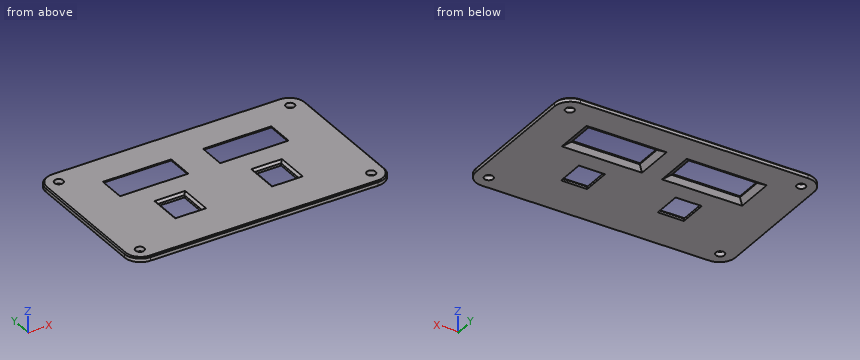
from build123d import *
from OCP.BRepFilletAPI import BRepFilletAPI_MakeChamfer

# Parameters (mm, degrees)
SKETCH1_R           = 1.9
BOSS_EXTRUDE1_DEPTH = 2
SKETCH6_W           = 11.5
SKETCH6_H           = 12.5
SKETCH6_W_2         = 30
SKETCH6_H_2         = 12
CUT_EXTRUDE2_DEPTH  = 2
CHAMFER4_SIZE       = 1
CHAMFER5_SIZE       = 1.5
CHAMFER5_SIZE2      = 2.598076211
CHAMFER6_SIZE       = 0.5


with BuildPart() as part:
    # Sketch1 → Boss-Extrude1 (new body)
    with BuildSketch(Plane.XY):
        with BuildLine():
            Line((-57, 27.5), (-57, -27.5))
            ThreePointArc((-57, -27.5), (-54.949747468, -32.449747468), (-50, -34.5))
            Line((-50, -34.5), (50, -34.5))
            ThreePointArc((50, -34.5), (54.949747468, -32.449747468), (57, -27.5))
            Line((57, -27.5), (57, 27.5))
            ThreePointArc((57, 27.5), (54.949747468, 32.449747468), (50, 34.5))
            Line((50, 34.5), (-50, 34.5))
            ThreePointArc((-50, 34.5), (-54.949747468, 32.449747468), (-57, 27.5))
        make_face()
        with Locations((-50.814035536, 28.314035536)):
            Circle(SKETCH1_R, mode=Mode.SUBTRACT)
        with Locations((50.814035536, 28.314035536)):
            Circle(SKETCH1_R, mode=Mode.SUBTRACT)
        with Locations((50.814035536, -28.314035536)):
            Circle(SKETCH1_R, mode=Mode.SUBTRACT)
        with Locations((-50.814035536, -28.314035536)):
            Circle(SKETCH1_R, mode=Mode.SUBTRACT)
    extrude(amount=BOSS_EXTRUDE1_DEPTH)

    # Sketch6 → Cut-Extrude2 (cut)
    with BuildSketch(Plane.XY.offset(2)):
        with Locations((-21.25, -9.5)):
            Rectangle(SKETCH6_W, SKETCH6_H)
        with Locations((21.25, -9.5)):
            Rectangle(SKETCH6_W, SKETCH6_H)
        with Locations((-22, 13.5)):
            Rectangle(SKETCH6_W_2, SKETCH6_H_2)
        with Locations((22, 13.5)):
            Rectangle(SKETCH6_W_2, SKETCH6_H_2)
    extrude(amount=-CUT_EXTRUDE2_DEPTH, mode=Mode.SUBTRACT)

    # Chamfer4
    chamfer4_edges = [part.edges().sort_by_distance(p)[0] for p in [
        (27, -9.5, 2),
        (21.25, -3.25, 2),
        (15.5, -9.5, 2),
        (21.25, -15.75, 2),
        (-15.5, -9.5, 2),
        (-21.25, -3.25, 2),
        (-27, -9.5, 2),
        (-21.25, -15.75, 2),
    ]]
    chamfer(chamfer4_edges, length=CHAMFER4_SIZE)

    # Chamfer5: one chamfer whose edges measure the first distance from different faces: ONE call of the kernel's chamfer builder (chamfer() names one face for all edges)
    chamfer5_edges_1 = [part.edges().sort_by_distance(p)[0] for p in [
        (-7, 13.5, 0),
    ]]
    chamfer5_side_1 = [part.faces().sort_by_distance(p)[0] for p in [
        (-7, 13.5, 1),
    ]]
    chamfer5_edges_2 = [part.edges().sort_by_distance(p)[0] for p in [
        (-22, 7.5, 0),
    ]]
    chamfer5_side_2 = [part.faces().sort_by_distance(p)[0] for p in [
        (-22, 7.5, 1),
    ]]
    chamfer5_edges_3 = [part.edges().sort_by_distance(p)[0] for p in [
        (-37, 13.5, 0),
    ]]
    chamfer5_side_3 = [part.faces().sort_by_distance(p)[0] for p in [
        (-37, 13.5, 1),
    ]]
    chamfer5_edges_4 = [part.edges().sort_by_distance(p)[0] for p in [
        (-22, 19.5, 0),
    ]]
    chamfer5_side_4 = [part.faces().sort_by_distance(p)[0] for p in [
        (-22, 19.5, 1),
    ]]
    chamfer5_edges_5 = [part.edges().sort_by_distance(p)[0] for p in [
        (37, 13.5, 0),
    ]]
    chamfer5_side_5 = [part.faces().sort_by_distance(p)[0] for p in [
        (37, 13.5, 1),
    ]]
    chamfer5_edges_6 = [part.edges().sort_by_distance(p)[0] for p in [
        (22, 7.5, 0),
    ]]
    chamfer5_side_6 = [part.faces().sort_by_distance(p)[0] for p in [
        (22, 7.5, 1),
    ]]
    chamfer5_edges_7 = [part.edges().sort_by_distance(p)[0] for p in [
        (7, 13.5, 0),
    ]]
    chamfer5_side_7 = [part.faces().sort_by_distance(p)[0] for p in [
        (7, 13.5, 1),
    ]]
    chamfer5_edges_8 = [part.edges().sort_by_distance(p)[0] for p in [
        (22, 19.5, 0),
    ]]
    chamfer5_side_8 = [part.faces().sort_by_distance(p)[0] for p in [
        (22, 19.5, 1),
    ]]
    chamfer5 = BRepFilletAPI_MakeChamfer(part.part.solid().wrapped)
    for e in chamfer5_edges_1:
        chamfer5.Add(CHAMFER5_SIZE, CHAMFER5_SIZE2, e.wrapped, chamfer5_side_1[0].wrapped)  # the first distance lies on this face
    for e in chamfer5_edges_2:
        chamfer5.Add(CHAMFER5_SIZE, CHAMFER5_SIZE2, e.wrapped, chamfer5_side_2[0].wrapped)  # the first distance lies on this face
    for e in chamfer5_edges_3:
        chamfer5.Add(CHAMFER5_SIZE, CHAMFER5_SIZE2, e.wrapped, chamfer5_side_3[0].wrapped)  # the first distance lies on this face
    for e in chamfer5_edges_4:
        chamfer5.Add(CHAMFER5_SIZE, CHAMFER5_SIZE2, e.wrapped, chamfer5_side_4[0].wrapped)  # the first distance lies on this face
    for e in chamfer5_edges_5:
        chamfer5.Add(CHAMFER5_SIZE, CHAMFER5_SIZE2, e.wrapped, chamfer5_side_5[0].wrapped)  # the first distance lies on this face
    for e in chamfer5_edges_6:
        chamfer5.Add(CHAMFER5_SIZE, CHAMFER5_SIZE2, e.wrapped, chamfer5_side_6[0].wrapped)  # the first distance lies on this face
    for e in chamfer5_edges_7:
        chamfer5.Add(CHAMFER5_SIZE, CHAMFER5_SIZE2, e.wrapped, chamfer5_side_7[0].wrapped)  # the first distance lies on this face
    for e in chamfer5_edges_8:
        chamfer5.Add(CHAMFER5_SIZE, CHAMFER5_SIZE2, e.wrapped, chamfer5_side_8[0].wrapped)  # the first distance lies on this face
    add(Compound.cast(chamfer5.Shape()), mode=Mode.REPLACE)

    # Chamfer6
    chamfer6_edges = [part.edges().sort_by_distance(p)[0] for p in [
        (57, 0, 2),
        (54.949747468, 32.449747468, 2),
        (0, 34.5, 2),
        (-54.949747468, 32.449747468, 2),
        (-57, 0, 2),
        (-54.949747468, -32.449747468, 2),
        (0, -34.5, 2),
        (54.949747468, -32.449747468, 2),
    ]]
    chamfer(chamfer6_edges, length=CHAMFER6_SIZE)


solid = part.part
For this review, take the finished solid that the model builds, in its own axes (mm). Give positions to 0.01 mm unless a question says otherwise; leave off trailing zeros. Loops run counter-clockwise (first coordinate to the right, second up) from the corner with the lowest first, then second, coordinate; pieces in that order, holes last.
Item 1: Take a section at C-C, the plane x = 10.5. State the section outline as (y, z) points.
Item 2: Take a section at B-B, the plane y = 17. State the section outline as (x, z) points, and give its area (4 significant figures).
Item 3: Take a section at A-A, the plane x = -25.5. State the section outline as (y, z) points, and give its area (3 significant figures).
Item 4: For line 1 along X through (y, z) = (-10, 0.55); line 2 along X through (y, z) = (-10, 1.35); line 3 along Y through (x, z) = (33, 1.65), list the stretches that pass through material, from the lowest coordinate up.
Item 5: Take a section at D-D, the plane z = 0.35. Give the number of separate pieces and of enclosed holes in the cut face, and give its area (3 significant figures).
Item 6: Insertion check: pin 1 (0.6 mm diameter, centred on x = -24.5, z = 2, fed in from -Y). The pin has a flat end and moves straight along its axis. Give the tip position at first contact, or say it passes through.
Calculated:
1. outline: (-34.5, 0) - (4.9, 0) - (7.5, 1.5) - (7.5, 2) - (-34, 2) - (-34.5, 1.5) - close; (19.5, 1.5) - (22.1, 0) - (34.5, 0) - (34.5, 1.5) - (34, 2) - (19.5, 2) - close
2. outline: (-57, 0) - (-39.6, 0) - (-37, 1.5) - (-37, 2) - (-56.5, 2) - (-57, 1.5) - close; (-7, 1.5) - (-4.4, 0) - (4.4, 0) - (7, 1.5) - (7, 2) - (-7, 2) - close; (37, 1.5) - (39.6, 0) - (57, 0) - (57, 1.5) - (56.5, 2) - (37, 2) - close
2. area: 100.0 mm2
3. outline: (-34.5, 0) - (-15.75, 0) - (-15.75, 1) - (-16.75, 2) - (-34, 2) - (-34.5, 1.5) - close; (-3.25, 0) - (4.9, 0) - (7.5, 1.5) - (7.5, 2) - (-2.25, 2) - (-3.25, 1) - close; (19.5, 1.5) - (22.1, 0) - (34.5, 0) - (34.5, 1.5) - (34, 2) - (19.5, 2) - close
3. area: 83.9 mm2
4. line 1: x = -57 to -27, -15.5 to 15.5, 27 to 57
4. line 2: x = -57 to -27.35, -15.15 to 15.15, 27.35 to 57
4. line 3: y = -34.35 to 7.5, 19.5 to 34.35
5. separate pieces: 1
5. enclosed holes: 8
5. area: 6,400 mm2
6. pin 1: stops at y = -34.3
